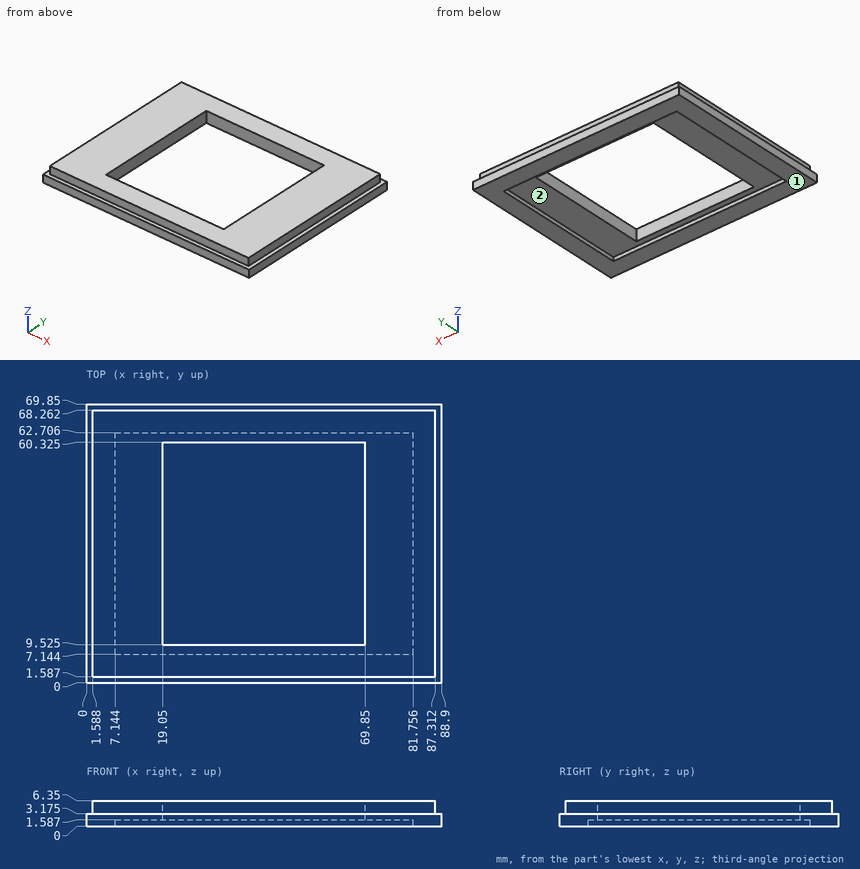
Drawing for the job (mm, zero at the part's lowest x, y, z). Give positions to 0.01 mm unless a question says otherwise; leave off trailing zeros. Write item = value, one per line. Start each with the question number.
1) Pull direction Y, two halves, no side cores. Call the marked faces 1 and 2: +Y half, -Y half, draft (parallel to the pull), parting line (faces both ways), or undercut.
2) Probe probe 1 along X at (y, z) = (23.5, 4); probe 2 along Y at (x, z) = (25, 4.75) (1 decimal); probe 3 along Y at (x, z) = (62.5, 1). List the from-to ranges inside material, lowest first. Write a range as from..to.
3) Drop flat-ended pins along their axis: pin 1 Ø3.5 at (x, z) = (44.5, 4.5) entering from +Y; pin 2 Ø2 at (y, z) = (50.5, 5) entering from -X; pin 3 Ø1.6 at (y, z) = (42.5, 5) entering from +X; pin 4 Ø1 at (x, z) = (30.5, 4.5) entering from -Y. Give the stop position or say it passes through.
Final values:
q1.face_1 = draft
q1.face_2 = undercut
q2.probe_1 = 1.59..19.05, 69.85..87.31
q2.probe_2 = 1.6..9.5, 60.3..68.3
q2.probe_3 = 0..7.14, 62.71..69.85
q3.pin_1 = 69.85
q3.pin_2 = 1.59
q3.pin_3 = 87.31
q3.pin_4 = 1.59
